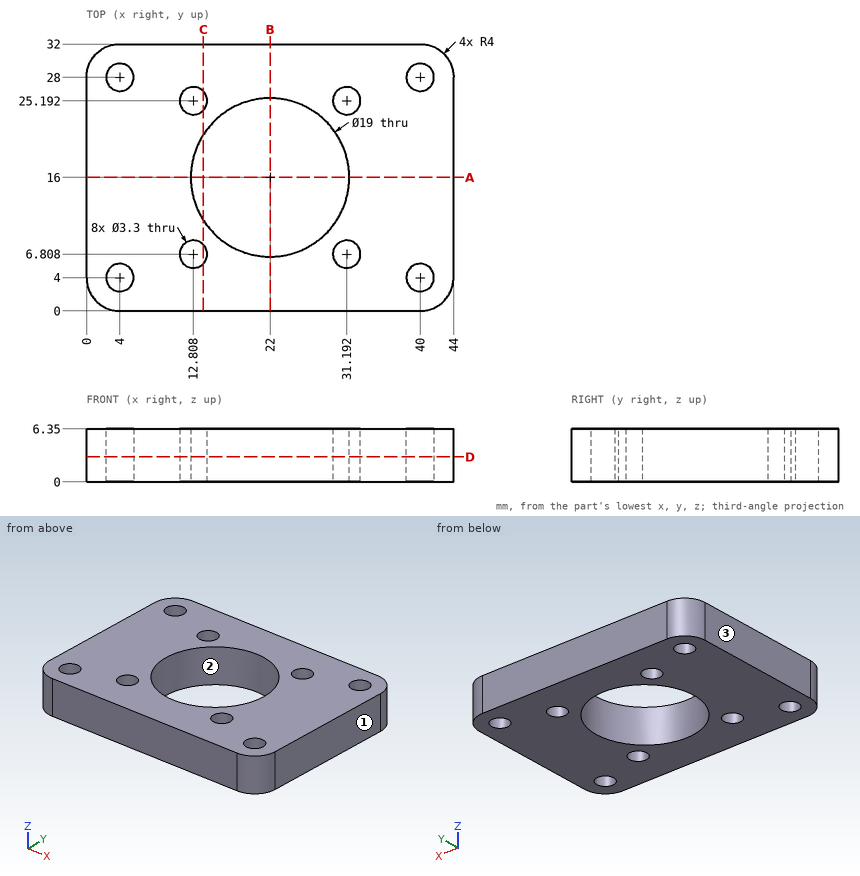
Source: three-view drawing plus pictorial views. Frame: mm from the lowest corner of the part. Coordinates: 2 decimals unless noted, no trailing zeros. Loops run counter-clockwise (first coordinate to the right, second up) from the corner with the lowest first, then second, coordinate; pieces in that order, holes last. Notation, with made-up numbers: (24, 51) -> (66, 51) arc R31 cw to (66, 77) -> close; hole circle Ø10 at (0, 62). An arc over 180 degrees is marked (long way). Write each question's results on one line, items separated by ' | '. Start each with the question number.
Q1. Section A-A, the plane y = 16. Return the cut outline in (x, z), plus the area to 3 significant figures.
Q2. Pull-direction query (X, two-part tool) for the marked faces 1, 2 and 3; classes: released by +X, released by -X, zero draft, split by the parting line, or undercut.
Q3. Section B-B, the plane x = 22. Return the cut outline in (y, z).
Q4. Ray query, line 1 (Y direction, x = 4, z = 5); line 2 (Y direction, x = 22, z = 4.25); line 3 (Y direction, x = 13.5, z = 5.75) (1 decimal). Return the intervals inside material, ascending. Write a range as from..to.
Q5. Pin query (flat end, axial travel): pin 1 (1 mm diameter, centred on x = 32, y = 19, fed in from -Z). Return the tip coordinate at first contact, or that it passes through.
Q6. Section C-C, the plane x = 14. Return the cut outline in (y, z).
Q7. Section D-D, the plane z = 3. State how many separate pieces and enclosed holes the cut face has, plus the area to 3 significant figures.
Found:
1) outline: (0, 0) -> (12.5, 0) -> (12.5, 6.35) -> (0, 6.35) -> close; (31.5, 0) -> (44, 0) -> (44, 6.35) -> (31.5, 6.35) -> close | area: 159 mm2
2) face 1: released by +X | face 2: undercut | face 3: released by -X
3) outline: (0, 0) -> (6.5, 0) -> (6.5, 6.35) -> (0, 6.35) -> close; (25.5, 0) -> (32, 0) -> (32, 6.35) -> (25.5, 6.35) -> close
4) line 1: 0..2.35, 5.65..26.35, 29.65..32 | line 2: 0..6.5, 25.5..32 | line 3: 0..5.3, 8.3..11.8, 20.2..23.7, 26.7..32
5) pin 1: z = 0
6) outline: (0, 0) -> (5.67, 0) -> (5.67, 6.35) -> (0, 6.35) -> close; (7.95, 0) -> (10.88, 0) -> (10.88, 6.35) -> (7.95, 6.35) -> close; (21.12, 0) -> (24.05, 0) -> (24.05, 6.35) -> (21.12, 6.35) -> close; (26.33, 0) -> (32, 0) -> (32, 6.35) -> (26.33, 6.35) -> close
7) separate pieces: 1 | enclosed holes: 9 | area: 1,040 mm2
